from build123d import *

# Parameters (mm, degrees)
KEEPER_START           = 0.55
SKETCH1_W              = 21.65
SKETCH1_H              = 9.6
KEEPER_DEPTH           = 5
BULKHEAD_START         = 0.35
BULKHEAD_CHAMFER_DEPTH = 5.4
TAB_START              = 0.35
SKETCH3_R              = 1.7
TAB_BOLT_HOLES_DEPTH   = 5.4
TAB_START_2            = 2.85
TAB_NUT_POCKETS_DEPTH  = 2.9


with BuildPart() as part:
    # Sketch1 → Keeper (new body)
    with BuildSketch(Plane(origin=(0, 0, 0), x_dir=(0, 0, -1), z_dir=(1, 0, 0)).offset(KEEPER_START)):
        with Locations((39.175, 117.7)):
            Rectangle(SKETCH1_W, SKETCH1_H)
    extrude(amount=KEEPER_DEPTH)

    # Sketch2 → Bulkhead chamfer (cut)
    with BuildSketch(Plane(origin=(0, 0, 0), x_dir=(0, 0, -1), z_dir=(1, 0, 0)).offset(BULKHEAD_START)):
        Polygon((21.8, 108.5), (21.8, 122.7), (30, 122.7), align=None)
    extrude(amount=BULKHEAD_CHAMFER_DEPTH, mode=Mode.SUBTRACT)

    # Sketch3 → Tab bolt holes (cut)
    with BuildSketch(Plane(origin=(0, 0, 0), x_dir=(0, 0, -1), z_dir=(1, 0, 0)).offset(TAB_START)):
        with Locations(Location((33.6, 116.9, 0), (0, 0, 180))):
            Circle(SKETCH3_R)
        with Locations(Location((43.6, 116.9, 0), (0, 0, 180))):
            Circle(SKETCH3_R)
    extrude(amount=TAB_BOLT_HOLES_DEPTH, mode=Mode.SUBTRACT)

    # Sketch4 → Tab nut pockets (cut)
    with BuildSketch(Plane(origin=(0, 0, 0), x_dir=(0, 0, -1), z_dir=(1, 0, 0)).offset(TAB_START_2)):
        Polygon((31.896816706, 119.85), (30.193633412, 116.9), (31.896816706, 113.95), (35.303183294, 113.95), (37.006366588, 116.9), (35.303183294, 119.85), align=None)
        Polygon((41.896816706, 119.85), (40.193633412, 116.9), (41.896816706, 113.95), (45.303183294, 113.95), (47.006366588, 116.9), (45.303183294, 119.85), align=None)
    extrude(amount=TAB_NUT_POCKETS_DEPTH, mode=Mode.SUBTRACT)


solid = part.part
Could you check a few things on this model? Use its own coordinates, in mm. A direction names the side the tool comes from. Give positions to 0.01 mm unless a question says otherwise; leave off trailing zeros. Order: outer loops, then holes, each group sorted by start corner. A loop starts at its lowest first (then second) coordinate and runs counter-clockwise, first axis right, second up.
Item 1: For faces 1 (the face through (4, 113.95, -44)), 2 (the face through (3, 112.9, -39)), which set-ups out of +Z, -Z, +X, -X, +Y, -Y let a thin tool reach every point of the face, with its end or its side?
Item 2: I need wall thicknesses on line 1 (Z direction, x = 1.75, y = 116.9); line 2 (Y direction, x = 1.25, z = -33.6); line 3 (Z direction, x = 4.75, y = 116). Which ranges of each line are inside material? Lowest first, please.
Item 3: If we mould it in two halves opening along Y, with no side actions, what happens to faces 3 (the face through (3, 118, -50)), 4 (the face through (4, 119.85, -44)), 5 (the face through (3.02, 121.19, -29.13))? For each: pulls with the +Y half, pulls with the -Y half, needs draft (parallel to the pull), parting line crosses it, or undercut.
Item 4: I'm going to push flat-ended pins straight in: pin 1 (1.8 mm diameter, centred on y = 116, z = -32, fed in from +X); pin 2 (4.5 mm diameter, centred on y = 116.9, z = -43.6, fed in from -X). Where does each tip first touch, or does it pass through?
Item 5: If we section it at C-C, the plane y = 118: Write out the boundary of the cut face in (x, z), plus the area to 3 significant figures.
Item 6: If we section it at D-D, the plane z = -36.25: Write out the boundary of the cut face in (x, y).
Item 7: If we section it at B-B, the plane z = -33.6: Write out the boundary of the cut face in (x, y), plus the area to 4 significant figures.
Item 8: If we section it at A-A, the plane x = 4.05: Write out the boundary of the cut face in (y, z).
Values:
1. face 1: +X
1. face 2: +Z, -Z, +X, -X, -Y
2. line 1: z = -50 to -45.3, -41.9 to -35.3, -31.9 to -28.35
2. line 2: y = 112.9 to 115.2, 118.6 to 122.5
2. line 3: z = -50 to -46.49, -40.71 to -36.49, -30.71 to -28.35
3. face 3: needs draft
3. face 4: undercut
3. face 5: pulls with the +Y half
4. pin 1: stops at x = 2.85
4. pin 2: stops at x = 0.55
5. outline: (0.55, -50) - (5.55, -50) - (5.55, -46.37) - (2.85, -46.37) - (2.85, -44.9) - (0.55, -44.9) - close; (0.55, -42.3) - (2.85, -42.3) - (2.85, -40.83) - (5.55, -40.83) - (5.55, -36.37) - (2.85, -36.37) - (2.85, -34.9) - (0.55, -34.9) - close; (0.55, -32.3) - (2.85, -32.3) - (2.85, -30.83) - (5.55, -30.83) - (5.55, -28.35) - (0.55, -28.35) - close
5. area: 66.4 mm2
6. outline: (0.55, 112.9) - (5.55, 112.9) - (5.55, 115.59) - (2.85, 115.59) - (2.85, 118.21) - (5.55, 118.21) - (5.55, 122.5) - (0.55, 122.5) - close
7. outline: (0.55, 112.9) - (5.55, 112.9) - (5.55, 113.95) - (2.85, 113.95) - (2.85, 115.2) - (0.55, 115.2) - close; (0.55, 118.6) - (2.85, 118.6) - (2.85, 119.85) - (5.55, 119.85) - (5.55, 122.5) - (0.55, 122.5) - close
7. area: 24.25 mm2
8. outline: (112.9, -50) - (122.5, -50) - (122.5, -29.88) - (119.84, -28.35) - (112.9, -28.35) - close; hole (113.95, -45.3) - (116.9, -47.01) - (119.85, -45.3) - (119.85, -41.9) - (116.9, -40.19) - (113.95, -41.9) - close; hole (113.95, -35.3) - (116.9, -37.01) - (119.85, -35.3) - (119.85, -31.9) - (116.9, -30.19) - (113.95, -31.9) - close
